Part print with two shaded views. Sizes in mm from the minimum x, y, z corner. Round coordinates to 2 decimals unless told otherwise and drop trailing zeros. Write each loop counter-clockwise with the first axis right and the second up, starting at its lowest first coordinate (ties: lowest second). Pieces come first, ordered by that corner, then holes. Notation, with made-up numbers: (-17, 70) -> (20, 70) arc R24 ccw to (20, 104) -> close; hole circle Ø4 at (13, 64.25). An arc over 180 degrees is marked (long way). Answer in a Markdown table with one row per item.
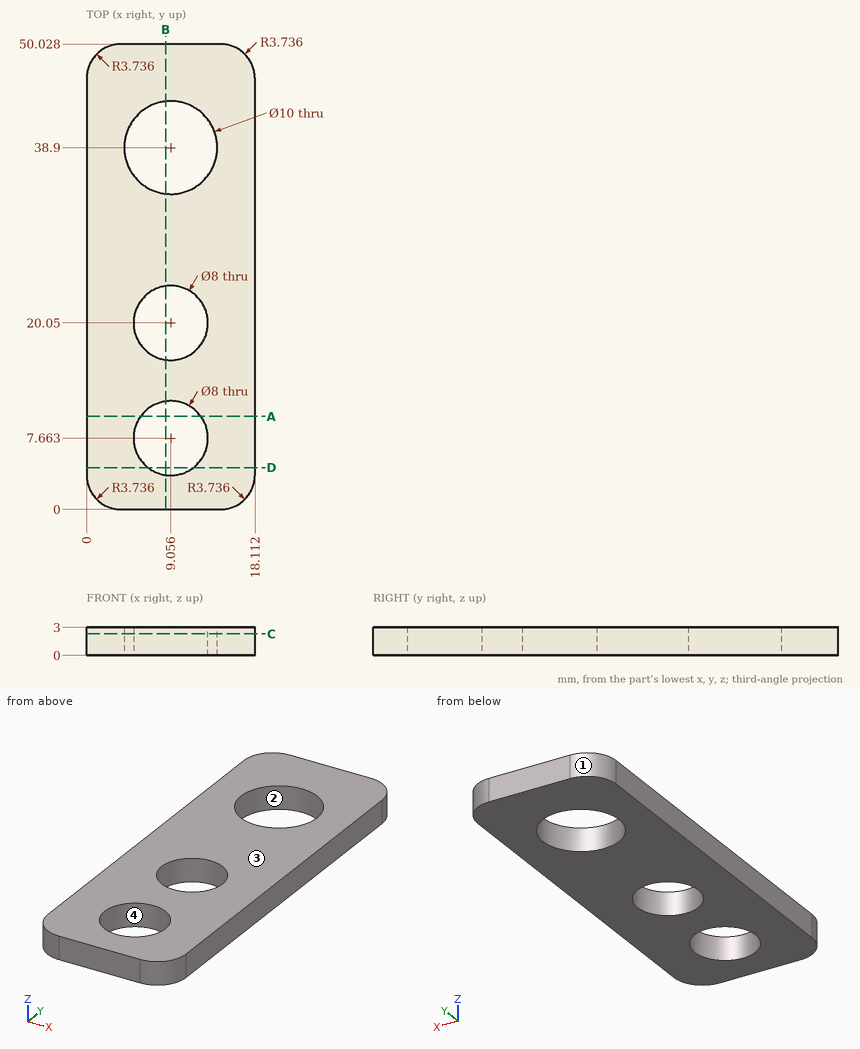
Q1. Saw through at D-D on y = 4.5. Write the cut outline in (x, z).
A:
| item | result |
|---|---|
| outline | (0, 0) -> (6.61, 0) -> (6.61, 3) -> (0, 3) -> close; (11.5, 0) -> (18.11, 0) -> (18.11, 3) -> (11.5, 3) -> close |
Q2. Two-plate mould, pull along Y, no slides. Class the marked faces 1, 2, 3 and 4: released by +Y, released by -Y, zero draft, split by the parting line, or undercut.
A:
| item | result |
|---|---|
| face 1 | released by +Y |
| face 2 | undercut |
| face 3 | zero draft |
| face 4 | undercut |
Q3. Saw through at C-C on z = 2.3. State how many separate pieces and enclosed holes the cut face has, plus the area to 3 significant figures.
A:
| item | result |
|---|---|
| separate pieces | 1 |
| enclosed holes | 3 |
| area | 715 mm² |
Q4. Wall check: line 1 (Y direction, x = 9, z = 1.1); line 2 (Y direction, x = 12.75, z = 1.55) (1 decimal); line 3 (X direction, y = 5, z = 1.4). Give the ranges that are in metal, low to high. Write a range as [from, to].
A:
| item | result |
|---|---|
| line 1 | [0, 3.66], [11.66, 16.05], [24.05, 33.9], [43.9, 50.03] |
| line 2 | [0, 6.1], [9.2, 18.5], [21.6, 35.5], [42.3, 50] |
| line 3 | [0, 6.07], [12.04, 18.11] |
Q5. Saw through at A-A on y = 10. Write the cut outline in (x, z).
A:
| item | result |
|---|---|
| outline | (0, 0) -> (5.81, 0) -> (5.81, 3) -> (0, 3) -> close; (12.3, 0) -> (18.11, 0) -> (18.11, 3) -> (12.3, 3) -> close |
Q6. Drop a flat-ended pin along its axis: P1, Ø6, axis at x = 9.06, y = 38.9, coming from the -Z side. Give the stop position or say it passes through.
A:
| item | result |
|---|---|
| P1 | through |
Q7. Saw through at B-B on x = 8.5. Write the cut outline in (y, z) (1 decimal).
A:
| item | result |
|---|---|
| outline | (0, 0) -> (3.7, 0) -> (3.7, 3) -> (0, 3) -> close; (11.6, 0) -> (16.1, 0) -> (16.1, 3) -> (11.6, 3) -> close; (24, 0) -> (33.9, 0) -> (33.9, 3) -> (24, 3) -> close; (43.9, 0) -> (50, 0) -> (50, 3) -> (43.9, 3) -> close |
